Geometry: see drawing. Coordinates: mm, zero at the bounding-box minimum. A direction names the side the tool comes from. Coordinates: 2 decimals unless noted, no trailing zeros. Loops run counter-clockwise (first coordinate to the right, second up) from the corner with the lowest first, then second, coordinate; pieces in that order, holes last. Notation, with made-up numbers: (17.25, 13) -> (26.25, 13) arc R21 ccw to (26.25, 35) -> close; hole circle Ø6 at (-39, -30). An arc over 180 degrees is marked (long way). One line per question, with ' | ' between items. Start each with the question number.
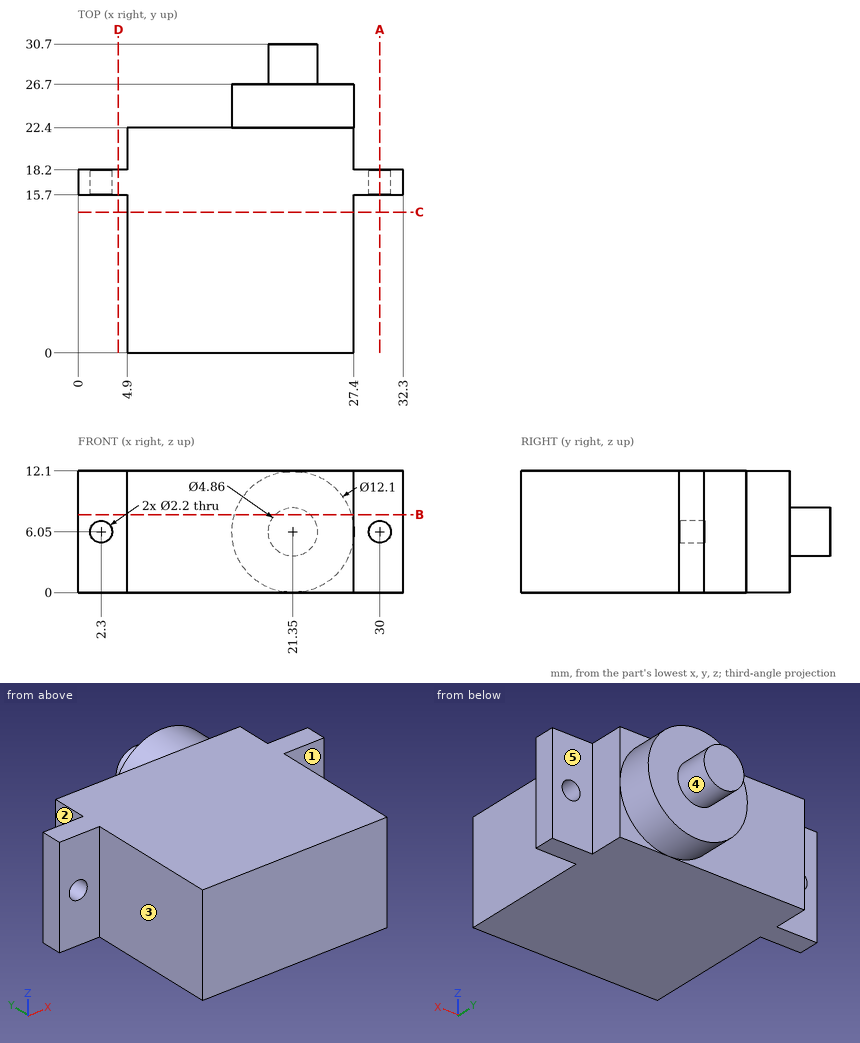
(1) Cut plane B-B, the plane z = 7.75. Return the cut outline in (x, y).
(2) Cut plane A-A, the plane x = 30. Return the cut outline in (y, z).
(3) Cut plane D-D, the plane x = 4. Return the cut outline in (y, z), and give its area (4 significant figures).
(4) Ray query, L1, parallel to X at y = 17.65, z = 6.05; L2, parallel to Y at x = 15, z = 2.75; L3, parallel to X at y = 6.5, z = 5.75. Return the intervals inside material, ascending.
(5) Cut plane C-C, the plane y = 14. Return the cut outline in (x, z).
(6) Contact query for flat-ended pins moving along their axis: pin 1 Ø1.5 at (x, z) = (31, 7) entering from +Y; pin 2 Ø6 at (y, z) = (7, 6.5) entering from +X; pin 3 Ø1.5 at (x, z) = (31, 5.5) entering from -Y. Output: stop coordinate, or through.
(7) Access query for the marked faces 1, 2, 3, 4 and 5. Directions: +Z, -Z, +X, -X, +Y, -Y. A direction counts if a zero-diameter tool reaches every point of the face in a straight line with its end or side. Return the directions, or none.
Here are the results:
1) outline: (0, 15.7) -> (4.9, 15.7) -> (4.9, 0) -> (27.4, 0) -> (27.4, 15.7) -> (32.3, 15.7) -> (32.3, 18.2) -> (27.4, 18.2) -> (27.4, 22.4) -> (27.16, 22.4) -> (27.16, 26.7) -> (23.09, 26.7) -> (23.09, 30.7) -> (19.61, 30.7) -> (19.61, 26.7) -> (15.54, 26.7) -> (15.54, 22.4) -> (4.9, 22.4) -> (4.9, 18.2) -> (0, 18.2) -> close
2) outline: (15.7, 0) -> (18.2, 0) -> (18.2, 4.95) -> (15.7, 4.95) -> close; (15.7, 7.15) -> (18.2, 7.15) -> (18.2, 12.1) -> (15.7, 12.1) -> close
3) outline: (15.7, 0) -> (18.2, 0) -> (18.2, 12.1) -> (15.7, 12.1) -> close | area: 30.25 mm2
4) L1: x = 0 to 1.2, 3.4 to 28.9, 31.1 to 32.3 | L2: y = 0 to 22.4 | L3: x = 4.9 to 27.4
5) outline: (4.9, 0) -> (27.4, 0) -> (27.4, 12.1) -> (4.9, 12.1) -> close
6) pin 1: stops at y = 18.2 | pin 2: stops at x = 27.4 | pin 3: stops at y = 15.7
7) face 1: +Z, -Z, +X, -Y | face 2: +Z, -Z, -X, +Y | face 3: +Z, -Z, -X, -Y | face 4: +Y | face 5: +Z, -Z, +X, +Y
